Could you check a few things on this model? Use its own coordinates, in mm. Face numbers are marked on the shaded views. A direction names the side the tool comes from. Round coordinates to 2 decimals unless told otherwise and drop trailing zeros. Loops run counter-clockwise (first coordinate to the right, second up) from the corner with the lowest first, then second, coordinate; pieces in that order, holes last. Notation, with made-up numbers: M -15,-1 L 18,-1 A29 ccw 18,27 Z; hole C 27,-23.75 d3. An arc over 180 degrees is marked long. One line per item, written item: value. Start each with the question number.
Q1. Which directions (+Z, -Z, +X, -X, +Y, -Y) give clear straight access to the entire face, cutting with the end or side of a thin tool? Please do the marked faces 5 and 6.
Q2. Imagine slicing it at D-D (x = 75.75). Please give me the cut outline in (y, z).
Q3. Please list where these lines run through material, in increasing order: line 1 along X through (y, z) = (197, -33.5); line 2 along Y through (x, z) = (75.75, -35.5); line 3 along X through (y, z) = (204.75, -35.75).
Q4. Imagine slicing it at C-C (z = -38.25). Please give me the cut outline in (x, y), then the cut area to 3 significant figures.
Q5. Imagine slicing it at A-A (y = 200). Please give me the cut outline in (x, z), then the cut area to 3 significant figures.
Q6. Thinking about a two-plate mould opening in Z: for the marked faces 1, 2, 3 and 4, which applies, released by +Z, released by -Z, zero draft, split by the parting line, or undercut?
Q7. Imagine slicing it at B-B (x = 82.75). Please give me the cut outline in (y, z), then the cut area to 3 significant figures.
Q8. I'm going to push flat-ended pins straight in: pin 1 Ø1.5 at (x, y) = (83, 205) entering from -Z; pin 2 Ø6 at (y, z) = (200, -33.5) entering from -X; pin 3 Ø8 at (x, y) = (76.5, 204.5) entering from +Z; pin 4 Ø5 at (x, y) = (84.5, 204) entering from -Z. Where does each tip first touch, or does it pass through?
from build123d import *

# Parameters (mm, degrees)
EXTRUDE_1_DEPTH                = 6
SKETCH_2_W                     = 12
SKETCH_2_H                     = 5.2
HOLE_WIZARD_M3_5_1_D           = 4
HOLE_WIZARD_M3_5_1_CBORE_D     = 5
HOLE_WIZARD_M3_5_1_CBORE_DEPTH = 12
SKETCH_5_W                     = 1.5
SKETCH_5_H                     = 6.915054242


with BuildPart() as part:
    # 草图1 → 凸台-拉伸1 (new body)
    with BuildSketch(Plane(origin=(88, 0, 0), x_dir=(0, 0, -1), z_dir=(1, 0, 0))):
        Polygon((27.096784191, 197.354470317), (32.589488008, 193.131887602), (38.992703817, 195.777417285), (39.903215809, 202.645529683), (34.410511992, 206.868112398), (28.007296183, 204.222582715), align=None)
    extrude(amount=-EXTRUDE_1_DEPTH)

    # 草图2 → 旋转1 (revolve)
    with BuildSketch(Plane.XY.offset(-33.5), mode=Mode.PRIVATE) as revolve_1_sk:
        with Locations((76, 202.6)):
            Rectangle(SKETCH_2_W, SKETCH_2_H)
    revolve(revolve_1_sk.sketch.rotate(Axis((70, 200, -33.5), (1, 0, 0)), 270), axis=Axis((70, 200, -33.5), (1, 0, 0)))

    # M3.5 六角头机械螺钉的柱形沉头孔1 (through all)
    with Locations(Plane.ZY.offset(-70)):
        with Locations((-33.5, 200)):
            CounterBoreHole(HOLE_WIZARD_M3_5_1_D / 2, HOLE_WIZARD_M3_5_1_CBORE_D / 2, HOLE_WIZARD_M3_5_1_CBORE_DEPTH)

    # 草图5 → Ø3.0 (3) 直径孔1 (revolve, cut)
    with BuildSketch(Plane(origin=(74, 198.322079162, -34.356128365), x_dir=(0, -0.3818493186865922, 0.9242245927363032), z_dir=(1, 0, 0))):
        with Locations((0.75, 3.457527121)):
            Rectangle(SKETCH_5_W, SKETCH_5_H)
    revolve(axis=Axis((74, 204.190905326, -31.931385192), (0, -0.9242245927363031, -0.38184931868659217)), mode=Mode.SUBTRACT)


solid = part.part
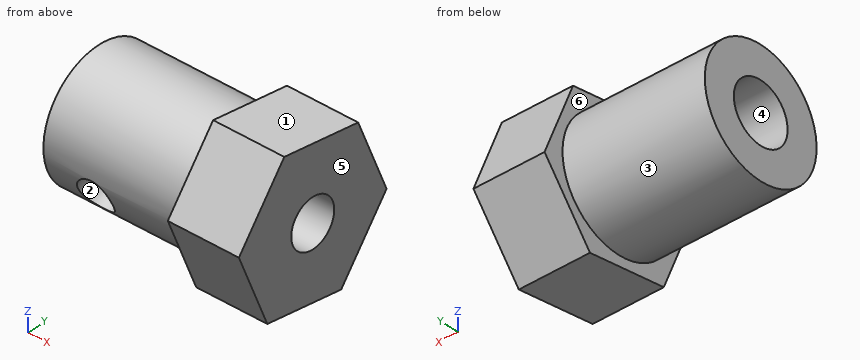
Report:
1. face 5: +Z, -Z, +X, +Y, -Y
1. face 6: -X
2. outline: C 200,-33.5 d10.4; hole C 200,-33.5 d5
3. line 1: x = 70 to 73.24, 74.76 to 88
3. line 2: y = 195.2 to 198.5, 201.5 to 204.8
3. line 3: x = 82 to 88
4. outline: M 70,197.88 L 82,197.88 L 82,195.47 L 88,195.47 L 88,203.92 L 82,203.92 L 82,202.12 L 70,202.12 Z
4. area: 101 mm²
5. outline: M 70,-38.7 L 82,-38.7 L 82,-39.55 L 88,-39.55 L 88,-35.5 L 82,-35.5 L 82,-36 L 70,-36 Z; M 70,-31 L 82,-31 L 82,-31.5 L 88,-31.5 L 88,-27.45 L 82,-27.45 L 82,-28.3 L 70,-28.3 Z
5. area: 113 mm²
6. face 1: released by +Z
6. face 2: undercut
6. face 3: split by the parting line
6. face 4: undercut
7. outline: M 193.13,-32.59 L 195.78,-38.99 L 202.65,-39.9 L 206.87,-34.41 L 204.22,-28.01 L 197.35,-27.1 Z; hole C 200,-33.5 d4
7. area: 112 mm²
8. pin 1: stops at z = -37.82
8. pin 2: stops at x = 70
8. pin 3: stops at z = -28.32
8. pin 4: stops at z = -39.9
